Autodesk Inventor part; units mm, degrees
ref_plane "YZ Plane" through (0, 0, 0) normal (1, 0, 0) x (0, 1, 0)
ref_plane "XZ Plane" through (0, 0, 0) normal (0, 1, 0) x (-1, 0, 0)
ref_plane "XY Plane" through (0, 0, 0) normal (0, 0, 1) x (1, 0, 0)
sketch "Эскиз1" plane through (0, 0, 0) normal (0, 1, 0) x (-1, 0, 0)
  line L0 (-15, 7.4) -> (15, 7.4)
  line L1 (15, 7.4) -> (15, -7.4)
  line L2 (15, -7.4) -> (-15, -7.4)
  line L3 (-15, -7.4) -> (-15, 7.4)
  line L4 (-15, 7.4) -> (15, -7.4) construction
  line L5 (15, 7.4) -> (-15, -7.4) construction
  point P0 (0, 0)
  dimension "d0" = 30
  dimension "d1" = 14.8
extrude "Выдавливание1" add sketch "Эскиз1" along normal mid plane 3.65
sketch "Эскиз2" plane through (0, -1.825, 0) normal (0, -1, 0) x (1, 0, 0)
  line L0 (-15, 7.4) -> (15, 7.4)
  line L1 (8.35, 7.4) -> (-8.35, 7.4)
  line L2 (-8.35, 7.4) -> (-8.35, 0.8)
  line L3 (-8.35, 0.8) -> (8.35, 0.8)
  line L4 (8.35, 0.8) -> (8.35, 7.4)
  point P0 (0, 0)
  point P1 (0, 7.4)
  dimension "d4" = 16.7
  dimension "d5" = 6.6
extrude "Выдавливание2" add sketch "Эскиз2" against normal blind 4.7
sketch "Эскиз3" plane through (0, 1.825, 0) normal (0, 1, 0) x (1, 0, 0)
  line L0 (15, -7.4) -> (-15, -7.4)
  line L1 (-15, -7.4) -> (-15, 7.4)
  line L2 (-15, 7.4) -> (15, 7.4)
  line L3 (15, 7.4) -> (15, -7.4)
  line L4 (13, -5.5) -> (-13, -5.5)
  line L5 (-13, -5.5) -> (-13, 5.5)
  line L6 (-13, 5.5) -> (13, 5.5)
  line L7 (13, 5.5) -> (13, -5.5)
  line L8 (13, -5.5) -> (-13, 5.5) construction
  line L9 (-13, -5.5) -> (13, 5.5) construction
  circle A0 centre (-13, -5.5) radius 1
  circle A1 centre (-13, 5.5) radius 1
  circle A2 centre (13, 5.5) radius 1
  circle A3 centre (13, -5.5) radius 1
  point P0 (0, 0)
  dimension "d8" = 26
  dimension "d9" = 11
  dimension "d10" = 2
  dimension "d11" = 2
  dimension "d12" = 2
  dimension "d13" = 2
extrude "Выдавливание3" cut sketch "Эскиз3" against normal blind 10 contours A0 L5 L4 | L4 L5 A0 | A3 L7 L4 | L4 L7 A3 | A1 L6 L5 | L5 L6 A1 | A2 L6 L7 | L7 L6 A2
properties part number "usb_camera_board"
The listing builds one solid part. Answer for the finished solid, in the listing's coordinates (mm). A direction names the side the tool comes from. Coordinates: 2 decimals unless noted, no trailing zeros. Order: outer loops, then holes, each group sorted by start corner. A loop starts at its lowest first (then second) coordinate and runs counter-clockwise, first axis right, second up. Notation, with made-up numbers: M 30,7.5 L 35,7.5 A23 cw 35,35.5 Z; hole C 47,70 d2. An arc over 180 degrees is marked long. Use CSV: the item, a comma, the result in double quotes.
Q1. Section D-D (z = 4) is taken. Determine the outline of the cut face in (x, y) (3 decimals).
Here are the results:
outline,"M -15,-1.825 L 15,-1.825 L 15,1.825 L 8.35,1.825 L 8.35,2.875 L -8.35,2.875 L -8.35,1.825 L -15,1.825 Z"
Q2. Given pin 1 Ø0.8 at (y, z) = (2.5, 3.5) entering from +X; pin 2 Ø0.5 at (y, z) = (2.5, 5) entering from -X; pin 3 Ø2.5 at (x, z) = (-13, -5.5) entering from +Y (3 decimals); pin 4 Ø1.8 at (x, z) = (13, -5.5) entering from +Y, each flat-ended and moving along its own axis, determine where each tip first touches the part or whether it passes through.
Here are the results:
pin 1,"x = 8.35"
pin 2,"x = -8.35"
pin 3,"y = 1.825"
pin 4,"through"
Q3. Determine the mould class of faces 1 (the cylindrical face through (-13.13, 0.03, -6.49)), 2 (the flat face through (0, 1.825, -2)), 3 (the flat face through (0, 0, 7.4)), 4 (the cylindrical face through (-13.13, 0.03, 4.51)) for opening direction Z: pulls with the +Z half, pulls with the -Z half, needs draft (parallel to the pull), parting line crosses it, or undercut.
Here are the results:
face 1,"undercut"
face 2,"needs draft"
face 3,"pulls with the +Z half"
face 4,"undercut"
Q4. A tool of negligible diameter and unlimited length cuts with its end or side. For faces 5 (the flat face through (15, 0, 0)), 6 (the flat face through (8.35, 2, 4)), 7 (the flat face through (0, 2, 0.8)), 8 (the flat face through (-8.35, 2, 4)), from which of +Z, -Z, +X, -X, +Y, -Y can it reach the whole face along a straight path? Write none if from no direction.
Here are the results:
face 5,"+Z, -Z, +X, +Y, -Y"
face 6,"+Z, -Z, +X, +Y"
face 7,"-Z, +X, -X, +Y"
face 8,"+Z, -Z, -X, +Y"
Q5. Section A-A (z = -5.5) is taken. Determine the outline of the cut face in (x, y) (3 decimals).
Here are the results:
outline,"M -15,-1.825 L -14,-1.825 L -14,1.825 L -15,1.825 Z; M -12,-1.825 L 12,-1.825 L 12,1.825 L -12,1.825 Z; M 14,-1.825 L 15,-1.825 L 15,1.825 L 14,1.825 Z"
Q6. Straight lines are drawn through the part: L1, parallel to X at y = 0.95, z = -5.5; L2, parallel to Z at x = 13, y = 0.75; L3, parallel to Z at x = -12.25, y = 0.2. For each, find the intervals that lie inside material, in ascending order.
Here are the results:
L1,"-15 to -14, -12 to 12, 14 to 15"
L2,"-7.4 to -6.5, -4.5 to 4.5, 6.5 to 7.4"
L3,"-7.4 to -6.16, -4.84 to 4.84, 6.16 to 7.4"
Q7. Section B-B (x = 13) is taken. Determine the outline of the cut face in (y, z) (3 decimals), then the cut area to 3 significant figures.
Here are the results:
outline,"M -1.825,-7.4 L 1.825,-7.4 L 1.825,-6.5 L -1.825,-6.5 Z; M -1.825,-4.5 L 1.825,-4.5 L 1.825,4.5 L -1.825,4.5 Z; M -1.825,6.5 L 1.825,6.5 L 1.825,7.4 L -1.825,7.4 Z"
area,"39.4 mm2"
Q8. Section C-C (y = -0.1) is taken. Determine the outline of the cut face in (x, z), then the cut area to 3 significant figures.
Here are the results:
outline,"M -15,-7.4 L 15,-7.4 L 15,7.4 L -15,7.4 Z; hole C -13,-5.5 d2; hole C -13,5.5 d2; hole C 13,-5.5 d2; hole C 13,5.5 d2"
area,"431 mm2"
